Autodesk Fusion 360 part; units mm, degrees
sketch "Sketch1" plane through (0, 0, 0) normal (0, 0, 1) x (1, 0, 0)
  line L0 (0, 0) -> (41, 0)
  line L1 (41, 0) -> (41, 35)
  line L2 (41, 35) -> (0, 35)
  line L3 (0, 35) -> (0, 0)
  line L4 (0, 17.5) -> (41, 17.5) construction
  circle A0 centre (4.8, 24.5) radius 2.75
  circle A1 centre (4.8, 10.5) radius 2.75
  line L5 (4.8, 24.5) -> (4.8, 10.5) construction
  line L6 (2.05, 10.5) -> (4.8, 10.5) construction
  line L7 (41, 37.525) -> (65, 37.525)
  line L8 (65, 37.525) -> (65, -2.475)
  line L9 (65, -2.475) -> (41, -2.475)
  line L10 (41, -2.475) -> (41, 0)
  line L11 (51, 29.5) -> (51, 5.55) construction
  circle A2 centre (51, 29.5) radius 2.75
  circle A3 centre (51, 5.55) radius 2.75
  line L12 (65, 17.525) -> (51, 17.525) construction
  line L13 (41, 37.525) -> (41, 35)
  line L14 (0, 0) -> (0, -2.475)
  line L15 (0, -2.475) -> (41, -2.475)
  point P0 (2.05, 10.5)
  dimension "d1" = 41
  dimension "d2" = 35
  dimension "d3" = 14
  dimension "d7" = 40
  dimension "d8" = 10
  dimension "d9" = 5.5
  dimension "d10" = 14
  dimension "d11" = 5
  dimension "d12" = 23.95
  dimension "d13" = 4.8
  dimension "d14" = 5.5
extrude "Extrude1" add sketch "Sketch1" along normal blind 6
extrude "Extrude2" cut sketch "Sketch1" along normal blind 2.1 from surface at 2 contours L0 L1 L2 L3
equation "d3 = ( ( 9 + 19 ) / 2 ) * 1 mm"
equation "d12 = ( ( 17.5 + 30.4 ) / 2 ) * 1 mm"
equation "d15 = 2 mm + 2 mm + 2 mm"
Here's how the part is built. I have some questions about the finished solid (model axes, mm). A direction names the side the tool comes from. Give positions to 0.01 mm unless a question says otherwise; leave off trailing zeros. Loops run counter-clockwise (first coordinate to the right, second up) from the corner with the lowest first, then second, coordinate; pieces in that order, holes last. Notation, with made-up numbers: M 26.5,66 L 75.5,66 A17 ccw 75.5,90 Z; hole C 50,4 d8. An arc over 180 degrees is marked long. Use one line per item in the form item = value. Start each with the question number.
Q1. If we section it at A-A (y = 5.55): Write out the boundary of the cut face in (x, z), then the cut area to 3 significant figures.
Q2. Which directions (+Z, -Z, +X, -X, +Y, -Y) give clear straight access to the entire face, cutting with the end or side of a thin tool? Please do faces 4 (the flat face through (20, 0, 3)), 5 (the flat face through (21, 35, 1)), 6 (the cylindrical face through (2.053, 10.379, 5.037)).
Q3. I need wall thicknesses on line 1 along Y through (x, z) = (4.8, 5.35) (3 decimals); line 2 along Y through (x, z) = (51, 3.3) (3 decimals); line 3 along Z through (x, y) = (15.5, 27). Which ranges of each line are inside material? Lowest first, please.
Q4. Thinking about a two-plate mould opening in Y: for faces 1 (the flat face through (21, 35, 5)), 2 (the cylindrical face through (48.253, 29.379, 2.958)), 3 (the flat face through (20, 18, 4.1)), which applies, +Y half, -Y half, draft (parallel to the pull), parting line (faces both ways), or undercut?
Q5. Will these pins go through, and if not, where does the flat tip stop? pin 1 Ø0.6 at (x, z) = (20.5, 5) entering from +Y; pin 2 Ø1.7 at (x, z) = (21, 3) entering from +Y; pin 3 Ø3.5 at (x, y) = (4.8, 10.5) entering from -Z.
Q6. If we section it at B-B (x = 51): Write out the boundary of the cut face in (y, z) (3 decimals).
Q7. If we section it at D-D (y = 10.5): Write out the boundary of the cut face in (x, z).
Q8. If we section it at C-C (z = 3.15): Write out the boundary of the cut face in (x, y) (3 decimals), then the cut area to 3 significant figures.
Taken from the geometry:
q1.outline = M 0,0 L 48.25,0 L 48.25,6 L 0,6 L 0,4.1 L 41,4.1 L 41,2 L 0,2 Z; M 53.75,0 L 65,0 L 65,6 L 53.75,6 Z
q1.area = 271 mm^2
q2.face_4 = -X, +Y
q2.face_5 = +Z, -Z, -X, +Y
q2.face_6 = +Z, -Z
q3.line_1 = -2.475 to 7.75, 13.25 to 21.75, 27.25 to 35
q3.line_2 = -2.475 to 2.8, 8.3 to 26.75, 32.25 to 37.525
q3.line_3 = 0 to 2, 4.1 to 6
q4.face_1 = +Y half
q4.face_2 = undercut
q4.face_3 = draft
q5.pin_1 = 35
q5.pin_2 = 0
q5.pin_3 = through
q6.outline = M -2.475,0 L 2.8,0 L 2.8,6 L -2.475,6 Z; M 8.3,0 L 26.75,0 L 26.75,6 L 8.3,6 Z; M 32.25,0 L 37.525,0 L 37.525,6 L 32.25,6 Z
q7.outline = M 0,0 L 2.05,0 L 2.05,2 L 0,2 Z; M 0,4.1 L 2.05,4.1 L 2.05,6 L 0,6 Z; M 7.55,0 L 65,0 L 65,6 L 7.55,6 L 7.55,4.1 L 41,4.1 L 41,2 L 7.55,2 Z
q8.outline = M 0,-2.475 L 65,-2.475 L 65,37.525 L 41,37.525 L 41,0 L 0,0 Z; hole C 51,5.55 d5.5; hole C 51,29.5 d5.5
q8.area = 1,010 mm^2
